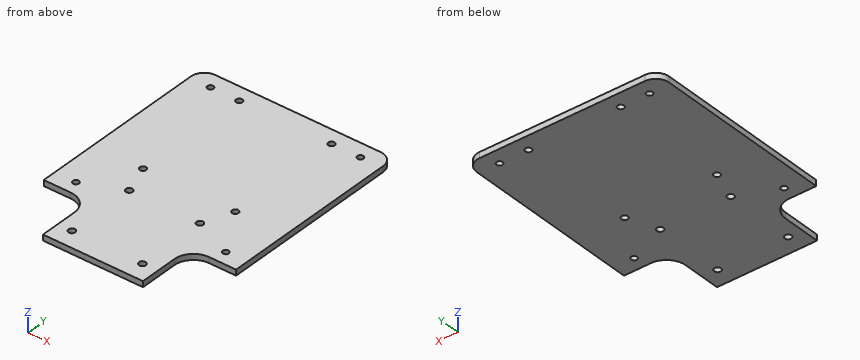
from build123d import *

# Parameters (mm, degrees)
SKETCH2_R           = 1.575
SKETCH2_R_2         = 1.75
BOSS_EXTRUDE1_DEPTH = 3
SKETCH3_R           = 1.65
CUT_EXTRUDE1_DEPTH  = 10
FILLET1_R           = 10


with BuildPart() as part:
    # Sketch2 → Boss-Extrude1 (new body)
    with BuildSketch(Plane.XY.offset(27)):
        with BuildLine():
            Line((50, 113.943914812), (50, 149))
            ThreePointArc((50, 149), (47.949747468, 153.949747468), (43, 156))
            Line((43, 156), (-43, 156))
            ThreePointArc((-43, 156), (-47.949747468, 153.949747468), (-50, 149))
            Line((-50, 149), (-50, 113.943914812))
            Line((-50, 113.943914812), (-50, 55))
            Line((-50, 55), (-26, 55))
            Line((-26, 55), (-26, 25))
            Line((-26, 25), (26, 25))
            Line((26, 25), (26, 55))
            Line((26, 55), (50, 55))
            Line((50, 55), (50, 113.943914812))
        make_face()
        with Locations((39, 62)):
            Circle(SKETCH2_R, mode=Mode.SUBTRACT)
        with Locations((-39, 62)):
            Circle(SKETCH2_R, mode=Mode.SUBTRACT)
        with Locations((39, 148)):
            Circle(SKETCH2_R, mode=Mode.SUBTRACT)
        with Locations((-39, 148)):
            Circle(SKETCH2_R, mode=Mode.SUBTRACT)
        with Locations((-18.621445193, 71.094788901)):
            Circle(SKETCH2_R_2, mode=Mode.SUBTRACT)
        with Locations((18.078554807, 71.094788901)):
            Circle(SKETCH2_R_2, mode=Mode.SUBTRACT)
        with Locations((-18.621445193, 34.394788901)):
            Circle(SKETCH2_R_2, mode=Mode.SUBTRACT)
        with Locations((18.078554807, 34.394788901)):
            Circle(SKETCH2_R_2, mode=Mode.SUBTRACT)
    extrude(amount=BOSS_EXTRUDE1_DEPTH)

    # Sketch3 → Cut-Extrude1 (cut)
    with BuildSketch(Plane.XY.offset(30)):
        with Locations((-24, 147.978654182)):
            Circle(SKETCH3_R)
        with Locations((24, 86.478654182)):
            Circle(SKETCH3_R)
        with Locations((-24, 86.478654182)):
            Circle(SKETCH3_R)
        with Locations((24, 147.978654182)):
            Circle(SKETCH3_R)
    extrude(amount=-CUT_EXTRUDE1_DEPTH, mode=Mode.SUBTRACT)

    # Fillet1
    fillet1_edges = [part.edges().sort_by_distance(p)[0] for p in [
        (26, 55, 28.5),
        (-26, 55, 28.5),
    ]]
    fillet(fillet1_edges, radius=FILLET1_R)


solid = part.part
Can you work these out from the model? Positions are in its coordinate system, mm. Give positions to 0.01 mm unless a question says otherwise; leave off trailing zeros. Order: outer loops, then holes, each group sorted by start corner. A loop starts at its lowest first (then second) coordinate and runs counter-clockwise, first axis right, second up. Notation, with made-up numbers: M 57,20.5 L 81,20.5 A6 cw 81,26.5 Z; hole C -11.75,26 d2. An arc over 180 degrees is marked long. One line per item, written item: value.
Item 1: If we section it at C-C on z = 28.45: State how many separate pieces and enclosed holes the cut face has, and give its area (3 significant figures).
Verdict:
separate pieces: 1
enclosed holes: 12
area: 11,600 mm2
Item 2: If we section it at D-D on y = 38.5: Write out the boundary of the cut face in (x, z), and give its area (3 significant figures).
Verdict:
outline: M -26,27 L 26,27 L 26,30 L -26,30 Z
area: 156 mm2
Item 3: Please list where these lines run through material, in increasing order: line 1 (Y direction, x = -39, z = 28) (3 decimals); line 2 (X direction, y = 148, z = 28.35) (3 decimals); line 3 (Y direction, x = 23.5, z = 29.1).
Verdict:
line 1: 55 to 60.425, 63.575 to 146.425, 149.575 to 156
line 2: -50 to -40.575, -37.425 to -25.65, -22.35 to 22.35, 25.65 to 37.425, 40.575 to 50
line 3: 25 to 84.91, 88.05 to 146.41, 149.55 to 156
Item 4: If we section it at A-A on y = 62: Write out the boundary of the cut face in (x, z) (3 decimals), and give its area (3 significant figures).
Verdict:
outline: M -50,27 L -40.575,27 L -40.575,30 L -50,30 Z; M -37.425,27 L 37.425,27 L 37.425,30 L -37.425,30 Z; M 40.575,27 L 50,27 L 50,30 L 40.575,30 Z
area: 281 mm2
Item 5: For pin 1 (3 mm diameter, centred on x = -18.62, y = 34.39, fed in from -Z); pin 2 (0.9 mm diameter, centred on x = 42, z = 28, fed in from -Y); pin 3 (0.9 mm diameter, centred on y = 33.5, z = 28.5, fed in from -X), each with a flat end and sliding along its axis, tell me the tip position at first contact or that it passes through.
Verdict:
pin 1: through
pin 2: y = 55
pin 3: x = -26
Item 6: If we section it at B-B on x = 24: Write out the boundary of the cut face in (y, z).
Verdict:
outline: M 25,27 L 84.83,27 L 84.83,30 L 25,30 Z; M 88.13,27 L 146.33,27 L 146.33,30 L 88.13,30 Z; M 149.63,27 L 156,27 L 156,30 L 149.63,30 Z
